Input: dimensioned drawing with shaded views. Units: mm. Origin: part minimum x, y, z. Round coordinates to 2 decimals unless told otherwise and drop trailing zeros. Loops run counter-clockwise (first coordinate to the right, second up) from the corner with the lowest first, then second, coordinate; pieces in that order, holes last.
1) Section A-A, the plane z = 5. Return loops of the section in (x, y), and give its area (3 significant figures).
2) Section C-C, the plane y = 141. Return loops of the section in (x, z).
3) Ray query, line 1 along X through (y, z) = (26.5, 5.25); line 2 along Y through (x, z) = (2.5, 6.75); line 3 along X through (y, z) = (102, 7). Return the intervals inside material, ascending.
4) Section B-B, the plane x = 5. Return loops of the section in (y, z), and give its area (3 significant figures).
5) First-contact query: pin 1 (2 mm diameter, centred on x = 3.5, z = 2, fed in from +Y); pin 2 (6 mm diameter, centred on y = 108, z = 5, fed in from +X); pin 3 (5 mm diameter, centred on x = 4, y = 111, fed in from -Z); pin 4 (3 mm diameter, centred on x = 3, y = 26, fed in from +Z). Flat tips, straight axial feed; report the tip coordinate or a pass-through.
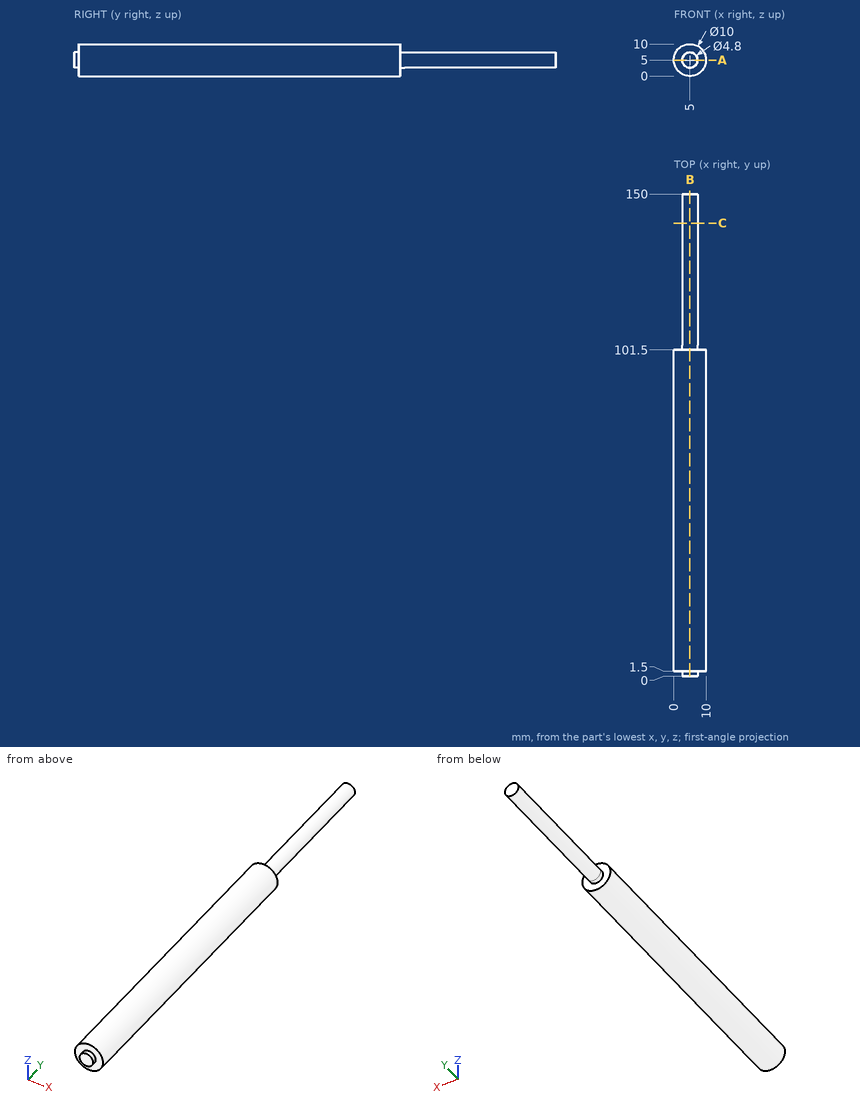
Final values:
1. outline: (0, 1.5) - (2.6, 1.5) - (2.6, 0) - (7.4, 0) - (7.4, 1.5) - (10, 1.5) - (10, 101.5) - (7.4, 101.5) - (7.4, 150) - (2.6, 150) - (2.6, 101.5) - (0, 101.5) - close
1. area: 1,240 mm2
2. outline: circle Ø4.8 at (5, 5)
3. line 1: x = 0.01 to 9.99
3. line 2: y = 1.5 to 101.5
3. line 3: x = 3.67 to 6.33
4. outline: (0, 2.6) - (1.5, 2.6) - (1.5, 0) - (101.5, 0) - (101.5, 2.6) - (150, 2.6) - (150, 7.4) - (101.5, 7.4) - (101.5, 10) - (1.5, 10) - (1.5, 7.4) - (0, 7.4) - close
4. area: 1,240 mm2
5. pin 1: stops at y = 150
5. pin 2: stops at x = 7.4
5. pin 3: stops at z = 2.6
5. pin 4: stops at z = 9.97
